Check sheet for the modelled part. Datum: model origin and axes. Units: mm. Face numbers are marked on the shaded views. Give positions to 0.01 mm unless a question says otherwise; leave off trailing zeros. Loops run counter-clockwise (first coordinate to the right, second up) from the corner with the lowest first, then second, coordinate; pieces in that order, holes last. Notation, with made-up numbers: (-22.5, 7.25) - (21.5, 7.25) arc R13 ccw to (21.5, 26.25) - close; hole circle Ø10 at (37, -31.5). An arc over 180 degrees is marked (long way). Use one line per item in the form item = value.
from build123d import *

# Parameters (mm, degrees)
SKETCH1_R           = 2.667
BOSS_EXTRUDE1_DEPTH = 11.43
CHAMFER1_SIZE       = 0.254
FILLET1_R           = 0.508


with BuildPart() as part:
    # Sketch1 → Boss-Extrude1 (new body)
    with BuildSketch(Plane(origin=(0, 0, 0), x_dir=(1, 0, 0), z_dir=(0, 1, 0))):
        Polygon((2.69097187, -4.6609), (5.381943739, 0), (2.69097187, 4.6609), (-2.69097187, 4.6609), (-5.381943739, 0), (-2.69097187, -4.6609), align=None)
        with Locations(Location((0, 0, 0), (0, 0, 270))):
            Circle(SKETCH1_R, mode=Mode.SUBTRACT)
    extrude(amount=BOSS_EXTRUDE1_DEPTH)

    # Chamfer1
    chamfer1_edges = [part.edges().sort_by_distance(p)[0] for p in [
        (4.036457804, 11.43, -2.33045),
        (0, 11.43, -4.6609),
        (-4.036457804, 11.43, -2.33045),
        (-4.036457804, 11.43, 2.33045),
        (0, 11.43, 4.6609),
        (-4.036457804, 0, 2.33045),
        (-4.036457804, 0, -2.33045),
        (0, 0, -4.6609),
        (4.036457804, 0, -2.33045),
        (4.036457804, 0, 2.33045),
        (0, 0, 4.6609),
        (4.036457804, 11.43, 2.33045),
    ]]
    chamfer(chamfer1_edges, length=CHAMFER1_SIZE)

    # Fillet1
    fillet1_edges = [part.edges().sort_by_distance(p)[0] for p in [
        (5.381943739, 5.715, 0),
        (2.69097187, 5.715, 4.6609),
        (2.69097187, 5.715, -4.6609),
        (-2.69097187, 5.715, -4.6609),
        (-5.381943739, 5.715, 0),
        (-2.69097187, 5.715, 4.6609),
    ]]
    fillet(fillet1_edges, radius=FILLET1_R)


solid = part.part
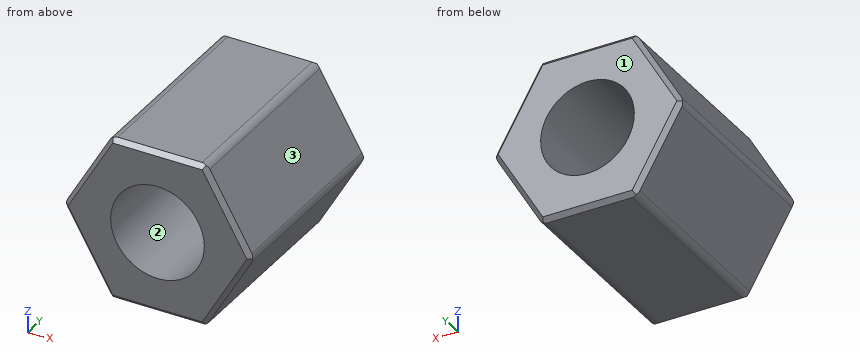
Item 1: Mould release check, pull along X, two halves, no side actions. Record for the marked faces 1, 2 and 3: released by +X, released by -X, zero draft, split by the parting line, or undercut.
Answer block:
face_1 = zero draft
face_2 = undercut
face_3 = released by +X
Item 2: Thickness scan on L1, parallel to X at y = 10.75, z = -1; L2, parallel to Z at x = 4, y = 10; L3, parallel to Z at x = -3, y = 5. Record the ranges inside material, lowest first.
Answer block:
L1 = -4.8 to -2.47, 2.47 to 4.8
L2 = -2.39 to 2.39
L3 = -4.13 to 4.13
Item 3: Section check A-A on x = 0. Record the boundary of the cut face in (y, z).
Answer block:
outline = (0, -4.41) - (0.25, -4.66) - (11.18, -4.66) - (11.43, -4.41) - (11.43, -2.67) - (0, -2.67) - close; (0, 2.67) - (11.43, 2.67) - (11.43, 4.41) - (11.18, 4.66) - (0.25, 4.66) - (0, 4.41) - close
Item 4: Gauge pin test, flat ends, axial feed: P1, Ø1.5, axis at x = 3.5, y = 4, coming from the -Z side; P2, Ø2, axis at y = 4, z = -2.5, coming from the +X side. Record the tip position at first contact, or that the pin passes through.
Answer block:
P1 = -4.52
P2 = 4.52
Item 5: Section check B-B on y = 4.75. Record the boundary of the cut face in (x, z), then the cut area to 3 significant figures.
Answer block:
outline = (-5.24, -0.25) - (-2.84, -4.41) arc R0.51 ccw to (-2.4, -4.66) - (2.4, -4.66) arc R0.51 ccw to (2.84, -4.41) - (5.24, -0.25) arc R0.51 ccw to (5.24, 0.25) - (2.84, 4.41) arc R0.51 ccw to (2.4, 4.66) - (-2.4, 4.66) arc R0.51 ccw to (-2.84, 4.41) - (-5.24, 0.25) arc R0.51 ccw to start; hole circle Ø5.33 at (0, 0)
area = 52.8 mm2
Item 6: Section check C-C on z = -1.75. Record the boundary of the cut face in (x, y), then the cut area to 3 significant figures.
Answer block:
outline = (-4.37, 0.25) - (-4.08, 0) - (-2.01, 0) - (-2.01, 11.43) - (-4.08, 11.43) - (-4.37, 11.18) - close; (2.01, 0) - (4.08, 0) - (4.37, 0.25) - (4.37, 11.18) - (4.08, 11.43) - (2.01, 11.43) - close
area = 53.8 mm2
Item 7: Section check D-D on z = -3.75. Record the boundary of the cut face in (x, y).
Answer block:
outline = (-3.22, 0.25) - (-2.92, 0) - (2.92, 0) - (3.22, 0.25) - (3.22, 11.18) - (2.92, 11.43) - (-2.92, 11.43) - (-3.22, 11.18) - close
